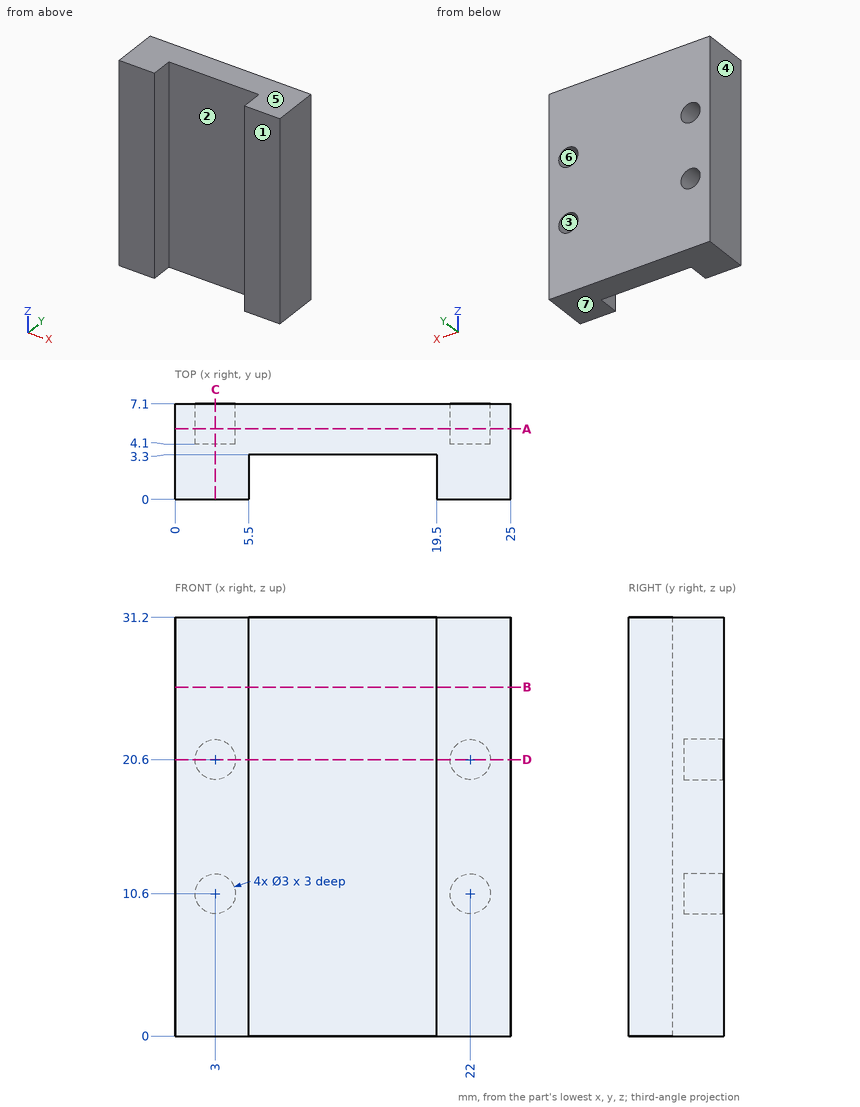
Input: dimensioned drawing with shaded views. Units: mm. Origin: part minimum x, y, z. A direction names the side the tool comes from. Round coordinates to 2 decimals unless told otherwise and drop trailing zeros. Loops run counter-clockwise (first coordinate to the right, second up) from the corner with the lowest first, then second, coordinate; pieces in that order, holes last. Notation, with made-up numbers: M -36,-24 L -10,-24 A14 cw -10,-16 Z; hole C 44,-32.75 d8. An arc over 180 degrees is marked long. One line per question, with ' | ' between items.
(1) Cut plane A-A on y = 5.25. Return the cut outline in (x, z), plus the area to 3 significant figures.
Check result:
outline: M 0,0 L 25,0 L 25,31.2 L 0,31.2 Z; hole C 3,10.6 d3; hole C 3,20.6 d3; hole C 22,10.6 d3; hole C 22,20.6 d3 | area: 752 mm2
(2) Contact query for flat-ended pins moving along their axis: P1, Ø2.5, axis at x = 3, z = 20.6, coming from the +Y side; P2, Ø4, axis at x = 12, z = 8.5, coming from the -Y side. Output: stop coordinate, or through.
Check result:
P1: stops at y = 4.1 | P2: stops at y = 3.3
(3) Cut plane B-B on z = 26. Return the cut outline in (x, y).
Check result:
outline: M 0,0 L 5.5,0 L 5.5,3.3 L 19.5,3.3 L 19.5,0 L 25,0 L 25,7.1 L 0,7.1 Z
(4) Access query for the marked faces 1, 2 and 3. Directions: +Z, -Z, +X, -X, +Y, -Y. A direction counts if a zero-diameter tool reaches every point of the face in a straight line with its end or side. Return the directions, or none.
Check result:
face 1: +Z, -Z, +X, -X, -Y | face 2: +Z, -Z, -Y | face 3: +Y
(5) Pull-direction query (Z, two-part tool) for the marked faces 4, 5, 6 and 7; classes: +Z half, -Z half, draft (parallel to the pull), parting line (faces both ways), or undercut.
Check result:
face 4: draft | face 5: +Z half | face 6: undercut | face 7: -Z half
(6) Cut plane C-C on x = 3. Return the cut outline in (y, z).
Check result:
outline: M 0,0 L 7.1,0 L 7.1,9.1 L 4.1,9.1 L 4.1,12.1 L 7.1,12.1 L 7.1,19.1 L 4.1,19.1 L 4.1,22.1 L 7.1,22.1 L 7.1,31.2 L 0,31.2 Z
(7) Material intervals for line 1 along X through (y, z) = (4.9, 20.6); line 2 along X through (y, z) = (3.25, 30.5); line 3 along Z through (x, y) = (22.25, 6.5), sorted ascending. Write a range as from..to.
Check result:
line 1: x = 0..1.5, 4.5..20.5, 23.5..25 | line 2: x = 0..5.5, 19.5..25 | line 3: z = 0..9.12, 12.08..19.12, 22.08..31.2
(8) Cut plane D-D on z = 20.6. Return the cut outline in (x, y).
Check result:
outline: M 0,0 L 5.5,0 L 5.5,3.3 L 19.5,3.3 L 19.5,0 L 25,0 L 25,7.1 L 23.5,7.1 L 23.5,4.1 L 20.5,4.1 L 20.5,7.1 L 4.5,7.1 L 4.5,4.1 L 1.5,4.1 L 1.5,7.1 L 0,7.1 Z
